Verification items for the finished model (mm, model axes). Coordinates: 2 decimals unless noted, no trailing zeros. Write each loop counter-clockwise with the first axis right and the second up, starting at its lowest first coordinate (ties: lowest second). Pieces come first, ordered by that corner, then holes. Notation, with made-up numbers: (-33.5, 75.25) -> (-17.5, 75.25) arc R21 ccw to (-17.5, 103.25) -> close; hole circle Ø9 at (53.5, -39.75). An arc over 180 degrees is marked (long way). Answer in a Markdown table with one row per item.
```python
from build123d import *

# Parameters (mm, degrees)
F0_R          = 4.7625
F1_DEPTH      = 25.4
F2_R          = 1.651
F3_DEPTH      = 4.7635
F3_DEPTH_BACK = 25.4
F4_R          = 1.27


with BuildPart() as f1:
    # F0 (on Top) → F1 (new body)
    with BuildSketch(Plane.XY):
        Circle(F0_R)
    extrude(amount=-F1_DEPTH)

    # F2 (on Front) → F3 (cut, two sides)
    with BuildSketch(Plane.XZ) as f3_sk:
        with Locations((0, -5.08)):
            Circle(F2_R)
    extrude(amount=-F3_DEPTH, mode=Mode.SUBTRACT)
    extrude(f3_sk.sketch, amount=F3_DEPTH_BACK, mode=Mode.SUBTRACT)

    # F4
    f4_edges = [f1.edges().sort_by_distance(p)[0] for p in [
        (-4.7625, 0, 0),
    ]]
    fillet(f4_edges, radius=F4_R)


solid = f1.part
```
1. Section check A-A, the plane x = 0. Record the boundary of the cut face in (y, z), plus the area to 3 significant figures.
Geometry says:
| item | result |
|---|---|
| outline | (-4.76, -25.4) -> (4.76, -25.4) -> (4.76, -6.73) -> (-4.76, -6.73) -> close; (-4.76, -3.43) -> (4.76, -3.43) -> (4.76, -1.27) arc R1.27 ccw to (3.49, 0) -> (-3.49, 0) arc R1.27 ccw to (-4.76, -1.27) -> close |
| area | 210 mm^2 |
2. Thickness scan on line 1 (Z direction, x = 0, y = 2.15); line 2 (X direction, y = 1.2, z = -5.08); line 3 (Z direction, x = -0.25, y = 4.25). Record the ranges inside material, lowest first. Write a range as from..to.
Geometry says:
| item | result |
|---|---|
| line 1 | -25.4..-6.73, -3.43..0 |
| line 2 | -4.61..-1.65, 1.65..4.61 |
| line 3 | -25.4..-6.71, -3.45..-0.26 |
3. Depth check by flat-ended pin: P1, Ø1.5, axis at x = -2.5, z = -16.5, coming from the -Y side; P2, Ø3, axis at x = -2.5, z = -3.5, coming from the +Y side; P3, Ø1.5, axis at y = 2.5, z = -21.5, coming from the -X side. Enter the tip coordinate at first touch or a pass-through.
Geometry says:
| item | result |
|---|---|
| P1 | y = -4.43 |
| P2 | y = 4.66 |
| P3 | x = -4.43 |
4. Section check B-B, the plane z = -5.5. Record the boundary of the cut face in (x, y) (1 decimal), plus the area to 3 significant figures.
Geometry says:
| item | result |
|---|---|
| outline | (-1.6, -4.5) -> (-1.6, 4.5) arc R4.8 ccw to start; (1.6, -4.5) arc R4.8 ccw to (1.6, 4.5) -> close |
| area | 41.4 mm^2 |
